CAD build for the part. Positions are in the model's coordinates, mm. A direction names the side the tool comes from. Round coordinates to 2 decimals unless told otherwise and drop trailing zeros. Write each loop counter-clockwise with the first axis right and the second up, starting at its lowest first coordinate (ties: lowest second). Pieces come first, ordered by that corner, then holes. Notation, with made-up numbers: (50, 89.5) - (78, 89.5) arc R32 ccw to (78, 121.5) - close; hole circle Ø4 at (-30.75, -10.5). An arc over 180 degrees is marked (long way). Put each result on its own line as item: value. Start each with the question number.
Item 1: Pin check, flat tips, straight feed: pin 1 Ø24 at (x, z) = (16.5, -74.5) entering from -Y; pin 2 Ø5 at (y, z) = (96, -7) entering from +X; pin 3 Ø19.5 at (y, z) = (100, 19) entering from +X. Stop position of each tip, or through.
Item 2: Cut at A-A (z = -80). Give the cut face in (x, y).
Item 3: Mould opens along Z. For faces 4 (the flat face through (-2.24, 65.829, 16.187)), 5 (the flat face through (10, 107, 15)), 6 (the flat face through (-40, 83, -68)), 7 (the cylindrical face through (36.99, 82.54, -97.15)) say: released by +Z, released by -Z, zero draft, split by the parting line, or undercut.
Item 4: Cut at C-C (z = 19). Give the cut face in (x, y).
Item 5: Drill centre lines: line 1 (X direction, y = 82, z = -80); line 2 (X direction, y = 82.95, z = -50); line 3 (Y direction, x = -17, z = 1). Where is each one in solid material? Low to high. Write a range as from..to.
Item 6: Cut at D-D (x = 25). Give the cut face in (y, z), and give its area (3 significant figures).
Item 7: 3-axis set-ups, long thin cutter, end or side, ignore diameter. For faces 1 (the cylindrical face through (0.21, 114.872, 20.953)), 2 (the flat face through (-1.5, 93, -9)), 3 (the flat face through (2.24, 96.392, -16.291)): which of +Z, -Z, +X, -X, +Y, -Y reach the whole face in a straight line?
Item 8: Cut at B-B (y = 100). Give the cut face in (x, z), and give its area (3 significant figures).
```python
from build123d import *

# Parameters (mm, degrees)
SKETCH1_R                    = 2.5
BASE_FLANGE1_DEPTH           = 5
SKETCH6_R                    = 2.5
BASE_FLANGE2_DEPTH           = 5
EDGE_FLANGE1_STRIP_W         = 24
EDGE_FLANGE1_STRIP_H         = 5
EDGE_FLANGE1_STRIP_CUT_DEPTH = 40
EDGE_FLANGE1_DEPTH           = 40
SKETCH19_R                   = 15
SKETCH19_R_2                 = 7.5
BOSS_EXTRUDE1_DEPTH          = 15
SKETCH20_R                   = 10
CUT_EXTRUDE1_DEPTH           = 5
BOSS_EXTRUDE2_DEPTH          = 3
CUT_EXTRUDE3_START           = 1.5
CUT_EXTRUDE3_DEPTH           = 1.5
CUT_EXTRUDE4_START           = 20
SKETCH23_R                   = 2.5
CUT_EXTRUDE4_DEPTH           = 126.187158898


# Sheet-metal steps are written as plain solids
with BuildPart() as part:
    # Sketch1 → Base-Flange1 (new body)
    with BuildSketch(Plane.XY):
        with BuildLine():
            Line((-30, 0), (30, 0))
            ThreePointArc((30, 0), (37.071067812, 2.928932188), (40, 10))
            Line((40, 10), (40, 35))
            Line((40, 35), (20, 58.835071852))
            Line((20, 58.835071852), (20, 85))
            Line((20, 85), (-20, 85))
            Line((-20, 85), (-20, 58.835071852))
            Line((-20, 58.835071852), (-40, 35))
            Line((-40, 35), (-40, 10))
            ThreePointArc((-40, 10), (-37.071067812, 2.928932188), (-30, 0))
        make_face()
        with Locations((17.5, 15)):
            Circle(SKETCH1_R, mode=Mode.SUBTRACT)
        with Locations((-17.5, 15)):
            Circle(SKETCH1_R, mode=Mode.SUBTRACT)
        with Locations((-17.5, 40)):
            Circle(SKETCH1_R, mode=Mode.SUBTRACT)
        with Locations((17.5, 40)):
            Circle(SKETCH1_R, mode=Mode.SUBTRACT)
    extrude(amount=BASE_FLANGE1_DEPTH)

    # Edge-Flange1 strip (across the edge) → Edge-Flange1 strip cut (cut)
    with BuildSketch(Plane(origin=(-20, 85, 0), x_dir=(0, -1, 0), z_dir=(1, 0, 0))):
        with Locations((-5, -2.5)):
            Rectangle(EDGE_FLANGE1_STRIP_W, EDGE_FLANGE1_STRIP_H)
    extrude(amount=EDGE_FLANGE1_STRIP_CUT_DEPTH, mode=Mode.SUBTRACT)

    # Edge-Flange1 section (across the edge) → Edge-Flange1 (add)
    with BuildSketch(Plane(origin=(-20, 85, 0), x_dir=(0, -1, 0), z_dir=(1, 0, 0))):
        with BuildLine():
            Line((0, 2), (0, 30.218007376))
            Line((0, 30.218007376), (5, 30.218007376))
            Line((5, 30.218007376), (5, 2))
            ThreePointArc((5, 2), (5.585786438, 0.585786438), (7, 0))
            Line((7, 0), (7, -5))
            ThreePointArc((7, -5), (2.050252532, -2.949747468), (0, 2))
        make_face()
    extrude(amount=EDGE_FLANGE1_DEPTH)


with BuildPart() as body_2:
    # Sketch6 → Base-Flange2 (new body)
    with BuildSketch(Plane(origin=(0, 85, 0), x_dir=(1, 0, 0), z_dir=(0, 1, 0))):
        with BuildLine():
            Line((-30, 100), (30, 100))
            ThreePointArc((30, 100), (37.071067812, 97.071067812), (40, 90))
            Line((40, 90), (40, 47))
            Line((40, 47), (20, 30.218007376))
            Line((20, 30.218007376), (-20, 30.218007376))
            Line((-20, 30.218007376), (-40, 47))
            Line((-40, 47), (-40, 90))
            ThreePointArc((-40, 90), (-37.071067812, 97.071067812), (-30, 100))
        make_face()
        with Locations(Location((-20, 80, 0), (0, 0, 270))):
            Circle(SKETCH6_R, mode=Mode.SUBTRACT)
        with Locations(Location((20, 80, 0), (0, 0, 90))):
            Circle(SKETCH6_R, mode=Mode.SUBTRACT)
        with Locations(Location((20, 51.246765298, 0), (0, 0, 270))):
            Circle(SKETCH6_R, mode=Mode.SUBTRACT)
        with Locations(Location((-20, 50, 0), (0, 0, 90))):
            Circle(SKETCH6_R, mode=Mode.SUBTRACT)
    extrude(amount=-BASE_FLANGE2_DEPTH)

    # Combine2: union part
    add(part.part)



with BuildPart() as body_2_2:
    # Sketch19 → Boss-Extrude1 (new, symmetric)
    with BuildSketch(Plane(origin=(0, 0, 0), x_dir=(0, 0, -1), z_dir=(1, 0, 0))):
        with Locations((-19, 100)):
            Circle(SKETCH19_R)
        with Locations((-19, 100)):
            Circle(SKETCH19_R_2, mode=Mode.SUBTRACT)
    extrude(amount=BOSS_EXTRUDE1_DEPTH, both=True)

    # Sketch20 → Cut-Extrude1 (cut)
    with BuildSketch(Plane(origin=(15, 0, 0), x_dir=(0, 0, -1), z_dir=(1, 0, 0))):
        with Locations((-19, 100)):
            Circle(SKETCH20_R)
    cut_extrude1 = extrude(amount=-CUT_EXTRUDE1_DEPTH, mode=Mode.SUBTRACT)

    # Mirror1: Cut-Extrude1 across plane
    add(cut_extrude1.mirror(Plane(origin=(0, 0, 0), x_dir=(0, 0, 1), z_dir=(1, 0, 0))), mode=Mode.SUBTRACT)


with BuildPart() as body_2_1:
    add(body_2.part)

    add(body_2_2.part)  # Boss-Extrude2 merges body 2 2
    # Sketch21 → Boss-Extrude2 (add, symmetric)
    with BuildSketch(Plane(origin=(0, 0, 0), x_dir=(0, 0, -1), z_dir=(1, 0, 0))):
        with BuildLine():
            Line((-32.573201875, 93.615002673), (-5, 35))
            Line((-5, 35), (-5, 78))
            ThreePointArc((-5, 78), (-2.949747468, 82.949747468), (2, 85))
            Line((2, 85), (47, 85))
            Line((47, 85), (-12.516699411, 113.526522593))
            ThreePointArc((-12.516699411, 113.526522593), (-8.431942873, 89.354993257), (-32.573201875, 93.615002673))
        make_face()
    extrude(amount=BOSS_EXTRUDE2_DEPTH, both=True)

    # Sketch22 → Cut-Extrude3 (cut)
    with BuildSketch(Plane(origin=(0, 0, 0), x_dir=(0, 0, -1), z_dir=(1, 0, 0)).offset(CUT_EXTRUDE3_START)):
        with BuildLine():
            Line((-24.147646276, 82.751761313), (-8, 48.425159203))
            Line((-8, 48.425159203), (-8, 85.752193151))
            ThreePointArc((-8, 85.752193151), (-15.711663212, 82.302914331), (-24.147646276, 82.751761313))
        make_face()
        with BuildLine():
            Line((33.8, 88), (-1.714869921, 105.02237774))
            ThreePointArc((-1.714869921, 105.02237774), (-1.447608596, 96.010820135), (-5.583592135, 88))
            Line((-5.583592135, 88), (33.8, 88))
        make_face()
    cut_extrude3 = extrude(amount=CUT_EXTRUDE3_DEPTH, mode=Mode.SUBTRACT)

    # Mirror4: Cut-Extrude3 across plane
    add(cut_extrude3.mirror(Plane(origin=(0, 0, 0), x_dir=(0, 0, 1), z_dir=(1, 0, 0))), mode=Mode.SUBTRACT)

    # Sketch23 → Cut-Extrude4 (cut, through all)
    with BuildSketch(Plane(origin=(20, 82.949747468, 2.949747468), x_dir=(1, 0, 0), z_dir=(0, 0.7071067811865468, 0.7071067811865483)).offset(CUT_EXTRUDE4_START)):
        with Locations(Location((-20, 0.707106781, 0), (0, 0, 90))):
            Circle(SKETCH23_R)
    extrude(amount=CUT_EXTRUDE4_DEPTH, mode=Mode.SUBTRACT)


solid = body_2_1.part
```
Output values:
1. pin 1: y = 80
1. pin 2: x = 1.5
1. pin 3: x = 10
2. outline: (-40, 80) - (-22.5, 80) - (-22.5, 85) - (-40, 85) - close; (-17.5, 80) - (17.5, 80) - (17.5, 85) - (-17.5, 85) - close; (22.5, 80) - (40, 80) - (40, 85) - (22.5, 85) - close
3. face 4: undercut
3. face 5: undercut
3. face 6: zero draft
3. face 7: released by -Z
4. outline: (-15, 85) - (-3, 85) - (-3, 82) - (-1.5, 82) - (-1.5, 71.81) - (-3, 71.81) - (-3, 64.76) - (3, 64.76) - (3, 71.81) - (1.5, 71.81) - (1.5, 82) - (3, 82) - (3, 85) - (15, 85) - (15, 90) - (10, 90) - (10, 92.5) - (-10, 92.5) - (-10, 90) - (-15, 90) - close; (-15, 110) - (-10, 110) - (-10, 107.5) - (10, 107.5) - (10, 110) - (15, 110) - (15, 115) - (-15, 115) - close
5. line 1: -40..-22.5, -17.5..17.5, 22.5..40
5. line 2: -40..-22.5, -17.5..17.83, 22.17..40
5. line 3: 0..12.55, 17.45..37.55, 42.45..84.32
6. outline: (0, 0) - (52.88, 0) - (52.88, 5) - (0, 5) - close; (80, -100) - (85, -100) - (85, -34.41) - (80, -34.41) - close
6. area: 592 mm2
7. face 1: none
7. face 2: -X
7. face 3: +X
8. outline: (-15, 4) - (-3, 4) - (-3, 1) - (-1.5, 1) - (-1.5, -8.76) - (-3, -8.76) - (-3, -15.7) - (3, -15.7) - (3, -8.76) - (1.5, -8.76) - (1.5, 1) - (3, 1) - (3, 4) - (15, 4) - (15, 9) - (10, 9) - (10, 11.5) - (-10, 11.5) - (-10, 9) - (-15, 9) - close; (-15, 29) - (-10, 29) - (-10, 26.5) - (10, 26.5) - (10, 29) - (15, 29) - (15, 34) - (-15, 34) - close
8. area: 489 mm2
